For this review, take the finished solid that the model builds, in its own axes (mm). Face numbers are marked on the shaded views. Give positions to 0.01 mm unless a question says otherwise; leave off trailing zeros. Order: outer loops, then holes, each group sorted by start corner. A loop starts at its lowest first (then second) coordinate and runs counter-clockwise, first axis right, second up.
from build123d import *

# Parameters (mm, degrees)
F0_W     = 35
F0_H     = 80
F0_R     = 4.25
F1_DEPTH = 10
F2_SIZE  = 5


with BuildPart() as f1:
    # F0 (on Front) → F1 (new body)
    with BuildSketch(Plane.XZ):
        Rectangle(F0_W, F0_H)
        with Locations((0, -22.25)):
            Circle(F0_R, mode=Mode.SUBTRACT)
        with Locations((0, 22.25)):
            Circle(F0_R, mode=Mode.SUBTRACT)
    extrude(amount=F1_DEPTH)

    # F2
    f2_edges = [f1.edges().sort_by_distance(p)[0] for p in [
        (-17.5, -5, 40),
        (17.5, -5, 40),
        (-17.5, -5, -40),
        (17.5, -5, -40),
    ]]
    chamfer(f2_edges, length=F2_SIZE)


solid = f1.part
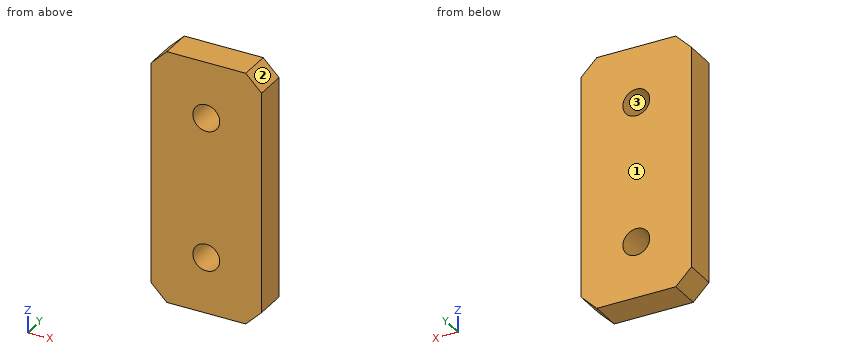
1) We need section D-D on z = 20. Give the boundary of the cut face in (x, y).
Answer sheet:
outline: (-17.5, -10) - (-3.61, -10) - (-3.61, 0) - (-17.5, 0) - close; (3.61, -10) - (17.5, -10) - (17.5, 0) - (3.61, 0) - close
2) Draft analysis for pull direction X (two halves, no side actions). For the marked faces 1, 2 and 3, state which applies: +X half, -X half, draft (parallel to the pull), parting line (faces both ways), or undercut.
Answer sheet:
face 1: draft
face 2: +X half
face 3: undercut
3) We need section B-B on z = -22.25. Give the boundary of the cut face in (x, y).
Answer sheet:
outline: (-17.5, -10) - (-4.25, -10) - (-4.25, 0) - (-17.5, 0) - close; (4.25, -10) - (17.5, -10) - (17.5, 0) - (4.25, 0) - close
4) We need section C-C on x = 0. Give the boundary of the cut face in (y, z).
Answer sheet:
outline: (-10, -40) - (0, -40) - (0, -26.5) - (-10, -26.5) - close; (-10, -18) - (0, -18) - (0, 18) - (-10, 18) - close; (-10, 26.5) - (0, 26.5) - (0, 40) - (-10, 40) - close
5) Clearance check with flat-ended pins moving along their axes: pin 1 (10 mm diameter, centred on x = 3.5, z = 24, fed in from -Y); pin 2 (5 mm diameter, centred on x = 0, z = 22.25, fed in from +Y). State where each tip first meets the part, or that it passes through.
Answer sheet:
pin 1: stops at y = -10
pin 2: passes through
6) To check wall thickness, follow line 1 (Z direction, x = 0, y = -5.5); line 2 (Z direction, x = 1.5, y = -2.25). State the ranges of each line that lie inside material, in increasing order.
Answer sheet:
line 1: z = -40 to -26.5, -18 to 18, 26.5 to 40
line 2: z = -40 to -26.23, -18.27 to 18.27, 26.23 to 40
7) We need section A-A on y = -4.75. Give the boundary of the cut face in (x, z).
Answer sheet:
outline: (-17.5, -35) - (-12.5, -40) - (12.5, -40) - (17.5, -35) - (17.5, 35) - (12.5, 40) - (-12.5, 40) - (-17.5, 35) - close; hole circle Ø8.5 at (0, -22.25); hole circle Ø8.5 at (0, 22.25)
